Geometry: see drawing. Coordinates: mm, zero at the bounding-box minimum. Give positions to 0.01 mm unless a question says otherwise; leave off trailing zeros. Order: outer loops, then holes, each group sorted by start corner. A loop starts at its lowest first (then second) coordinate and runs counter-clockwise, first axis right, second up. Notation, with made-up numbers: M 79.5,-7.75 L 134.5,-7.75 A24 cw 134.5,13.25 Z; hole C 68,86 d8. An arc over 180 degrees is marked long. Write item = value, one per line. Start each with the question number.
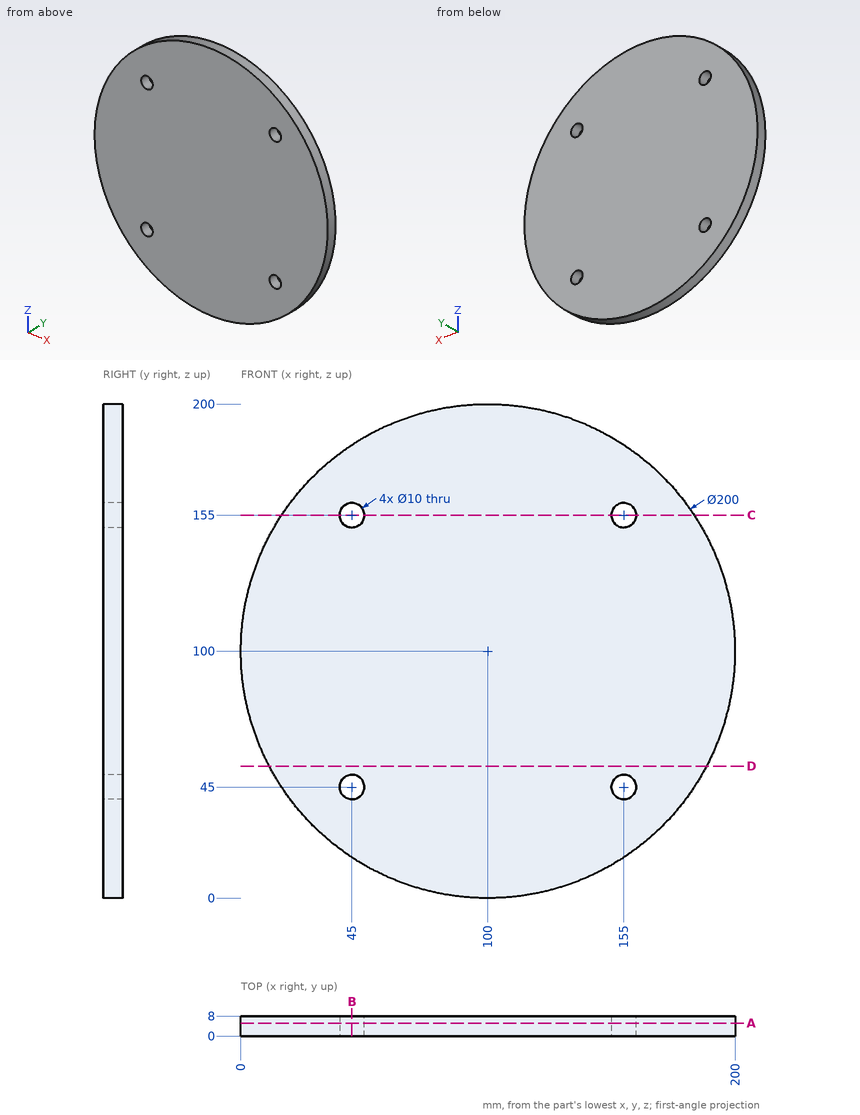
1) Pin query (flat end, axial travel): pin 1 Ø4 at (y, z) = (5, 87.5) entering from -X; pin 2 Ø9 at (x, z) = (45, 45) entering from -Y; pin 3 Ø6 at (x, z) = (25.5, 116.5) entering from -Y; pin 4 Ø1.5 at (x, y) = (86, 3) entering from +Z. Return the tip coordinate at first contact, or that it passes through.
2) Ray query, L1, parallel to X at y = 5.5, z = 45; L2, parallel to Z at x = 159.5, y = 5. Return the intervals inside material, ascending.
3) Cut plane C-C (z = 155). Return loops of the section in (x, y), plus the area to 3 significant figures.
4) Cut plane B-B (x = 45). Return loops of the section in (y, z).
5) Cut plane A-A (y = 5.25). Return loops of the section in (x, z).
6) Cut plane D-D (z = 53.5). Return loops of the section in (x, y), plus the area to 3 significant figures.
Reply:
q1.pin_1 = 0.55
q1.pin_2 = through
q1.pin_3 = 0
q1.pin_4 = 199.12
q2.L1 = 16.48 to 40, 50 to 150, 160 to 183.52
q2.L2 = 19.63 to 42.82, 47.18 to 152.82, 157.18 to 180.37
q3.outline = M 16.48,0 L 40,0 L 40,8 L 16.48,8 Z; M 50,0 L 150,0 L 150,8 L 50,8 Z; M 160,0 L 183.52,0 L 183.52,8 L 160,8 Z
q3.area = 1,180 mm²
q4.outline = M 0,16.48 L 8,16.48 L 8,40 L 0,40 Z; M 0,50 L 8,50 L 8,150 L 0,150 Z; M 0,160 L 8,160 L 8,183.52 L 0,183.52 Z
q5.outline = C 100,100 d200; hole C 45,45 d10; hole C 45,155 d10; hole C 155,45 d10; hole C 155,155 d10
q6.outline = M 11.47,0 L 188.53,0 L 188.53,8 L 11.47,8 Z
q6.area = 1,420 mm²
